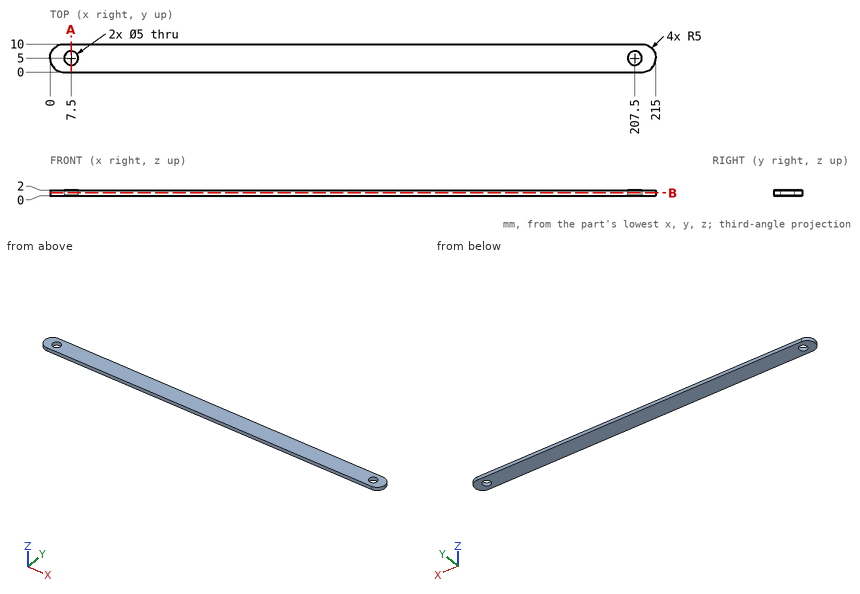
For this review, use the dimensioned drawing (mm, ordinates from the lowest corner) and the shaded views. Round coordinates to 2 decimals unless told otherwise and drop trailing zeros. Loops run counter-clockwise (first coordinate to the right, second up) from the corner with the lowest first, then second, coordinate; pieces in that order, holes last. Notation, with made-up numbers: M -8,-31 L 1,-31 A16 cw 1,-16 Z; hole C 88.25,57.25 d8. An arc over 180 degrees is marked long. Answer as a JSON object with one key per item and string values.
(1) Take a section at B-B on z = 1. Count the separate pieces of the cut face and the enclosed holes in it, and give its area (3 significant figures).
Resolved:
{"separate pieces": "1", "enclosed holes": "2", "area": "2,090 mm²"}
(2) Clearance check with flat-ended pins moving along their axes: P1, Ø1, axis at y = 2, z = 1, coming from the +X side; P2, Ø4, axis at x = 7.5, y = 5, coming from the -Z side. State where each tip first meets the part, or that it passes through.
Resolved:
{"P1": "x = 214.33", "P2": "through"}
(3) Take a section at A-A on x = 7.5. Give the boundary of the cut face in (y, z).
Resolved:
{"outline": "M 0,0 L 2.5,0 L 2.5,2 L 0,2 Z; M 7.5,0 L 10,0 L 10,2 L 7.5,2 Z"}
(4) To check wall thickness, follow line 1 along Y through (x, z) = (7.5, 0.75); line 2 along X through (y, z) = (3.75, 1.1) (1 decimal); line 3 along Y through (x, z) = (9, 0.85). State the ranges of each line that lie inside material, in increasing order.
Resolved:
{"line 1": "0 to 2.5, 7.5 to 10", "line 2": "0.2 to 5.3, 9.7 to 205.3, 209.7 to 214.8", "line 3": "0 to 3, 7 to 10"}
